Geometry: see drawing. Coordinates: mm, zero at the bounding-box minimum. Round coordinates to 2 decimals unless told otherwise and drop trailing zeros. Loops run counter-clockwise (first coordinate to the right, second up) from the corner with the lowest first, then second, coordinate; pieces in that order, holes last. Notation, with made-up numbers: (74, 86) - (118, 86) arc R11 ccw to (118, 99) - close; hole circle Ø6 at (50, -39.5). An arc over 180 degrees is marked (long way). Return JSON: item names as keys, results as strings. Group by question number.
1. Section C-C on y = 150. Return loops of the section in (x, z), and give its area (3 significant figures).
2. Section D-D on z = 1.5. Return loops of the section in (x, y).
3. First-contact query: pin 1 Ø4 at (x, y) = (5, 30) entering from -Z; pin 2 Ø6 at (x, y) = (5, 90) entering from -Z; pin 3 Ø5 at (x, y) = (6, 86) entering from +Z. Flat tips, straight axial feed; report the tip coordinate or a pass-through.
4. Section B-B on x = 5. Count the separate pieces of the cut face and the enclosed holes in it, and give its area (3 significant figures).
5. Section A-A on y = 70. Return loops of the section in (x, z).
6. Material intervals for probe 1 along Z at (x, y) = (8, 112); probe 2 along X at (y, z) = (130, 4.45); probe 3 along X at (y, z) = (8, 3.25), sorted ascending.
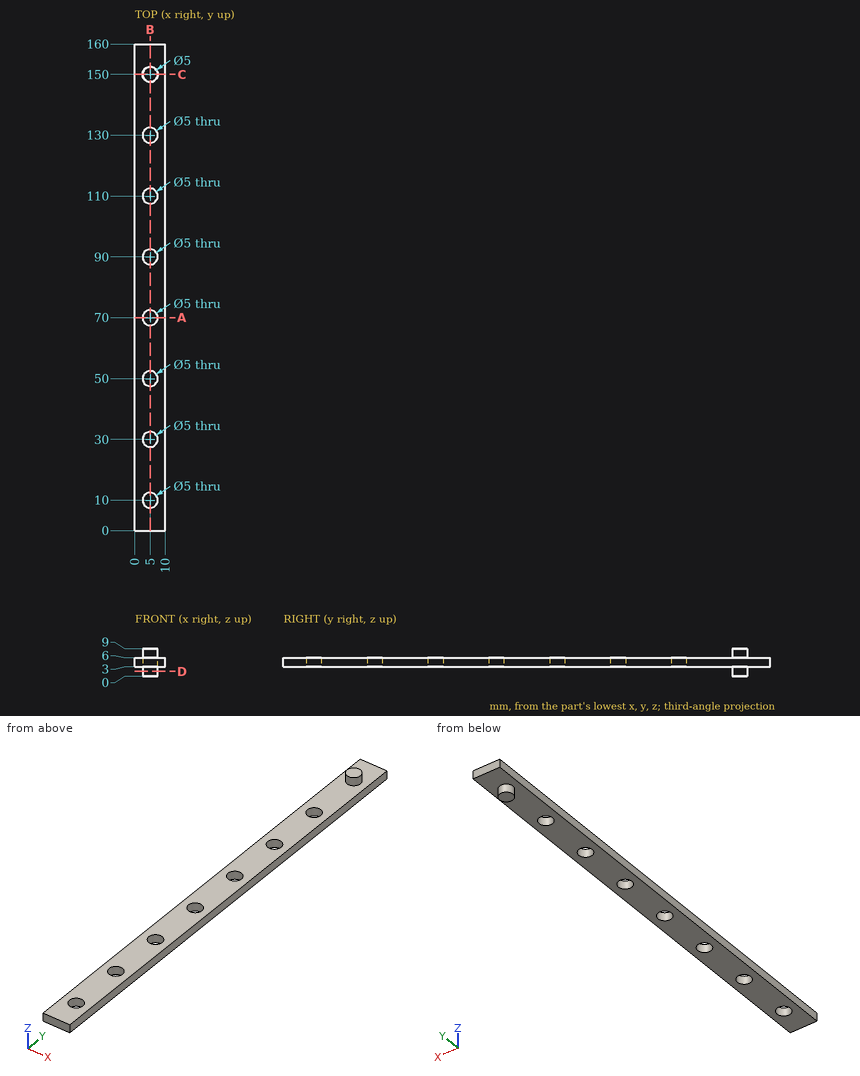
Taken from the geometry:
{
 "1": {"outline": "(0, 3) - (2.5, 3) - (2.5, 0) - (7.5, 0) - (7.5, 3) - (10, 3) - (10, 6) - (7.5, 6) - (7.5, 9) - (2.5, 9) - (2.5, 6) - (0, 6) - close", "area": "60.0 mm2"},
 "2": {"outline": "circle Ø5 at (5, 150)"},
 "3": {"pin 1": "through", "pin 2": "z = 3", "pin 3": "z = 6"},
 "4": {"separate pieces": "8", "enclosed holes": "0", "area": "405 mm2"},
 "5": {"outline": "(0, 3) - (2.5, 3) - (2.5, 6) - (0, 6) - close; (7.5, 3) - (10, 3) - (10, 6) - (7.5, 6) - close"},
 "6": {"probe 1": "3 to 6", "probe 2": "0 to 2.5, 7.5 to 10", "probe 3": "0 to 3.5, 6.5 to 10"}
}
